Job drawing, mm, ordinate dimensions from the low corner. One solid piece. A direction names the side the tool comes from. Coordinates: 2 decimals unless noted, no trailing zeros. Order: outer loops, then holes, each group sorted by start corner. A loop starts at its lowest first (then second) coordinate and runs counter-clockwise, first axis right, second up. Notation, with made-up numbers: M -7.75,83 L 42.25,83 A27 cw 42.25,99 Z; hole C -7,76.25 d8. An arc over 180 degrees is marked long. Write item = value, one per line. Start each with the question number.
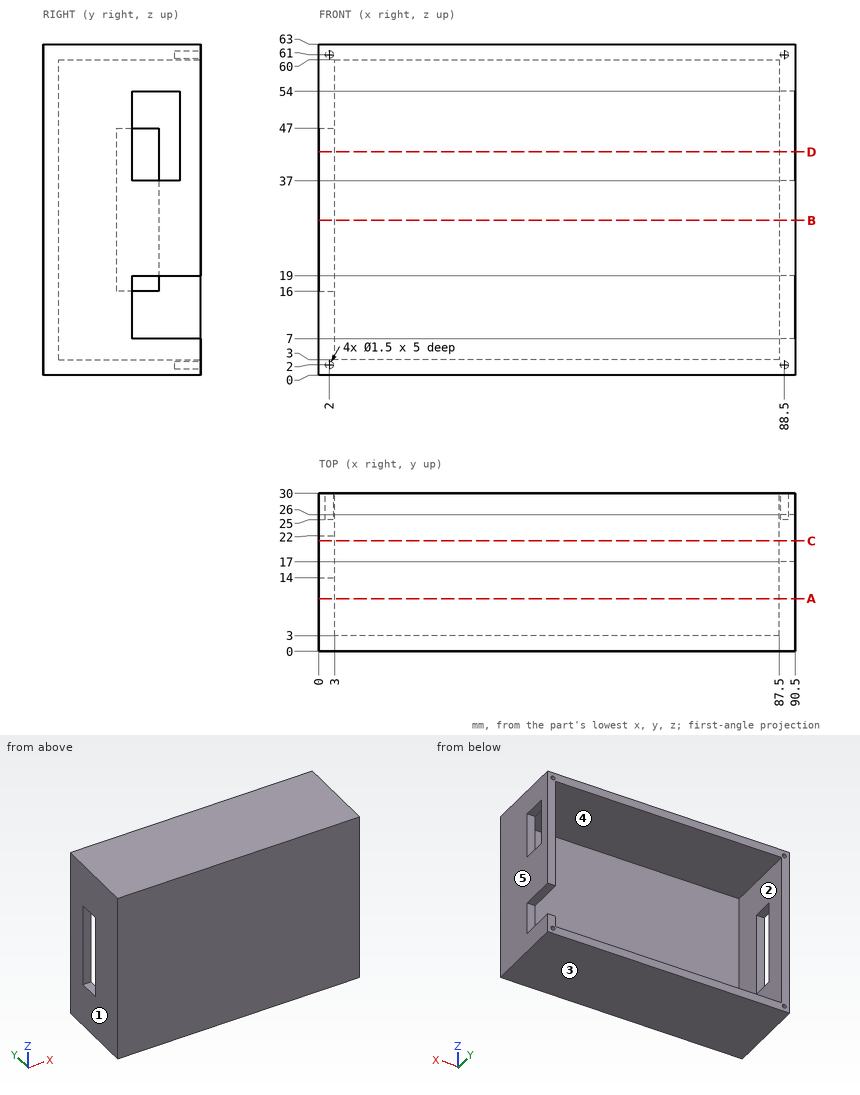
Item 1: Cut at D-D, the plane z = 42.5. Write the cut outline in (x, y).
Item 2: 3-axis set-ups, long thin cutter, end or side, ignore diameter. For the marked faces 4 and 5: which of +Z, -Z, +X, -X, +Y, -Y reach the whole face in a straight line?
Item 3: Wall check: line 1 along Z through (x, y) = (2, 27.75); line 2 along Z through (x, y) = (88.5, 26.65); line 3 along X through (y, z) = (28.85, 61). Give the ranges that are in metal, low to high. Write a range as [from, to].
Item 4: Cut at A-A, the plane y = 10. Write the cut outline in (x, z), and give its area (3 significant figures).
Item 5: Flat gauge pins, fed straight in: pin 1 (1.5 mm diameter, centred on x = 22.5, z = 24, fed in from -Y); pin 2 (1.2 mm diameter, centred on x = 2, z = 61, fed in from +Y); pin 3 (10 mm diameter, centred on x = 25, z = 43, fed in from +Y). Where does each tip first touch, or does it go through?
Item 6: Cut at B-B, the plane z = 29.5. Write the cut outline in (x, y), and give its area (4 significant figures).
Item 7: Cut at C-C, the plane y = 21. Write the cut outline in (x, z).
Item 8: Pull direction X, two halves, no side cores. Call the marked faces 1, 2 and 3: pulls with the +X half, pulls with the -X half, needs draft (parallel to the pull), parting line crosses it, or undercut.
Filled sheet:
q1.outline = M 0,0 L 90.5,0 L 90.5,17 L 87.5,17 L 87.5,3 L 3,3 L 3,14 L 0,14 Z; M 0,22 L 3,22 L 3,30 L 0,30 Z; M 87.5,26 L 90.5,26 L 90.5,30 L 87.5,30 Z
q2.face_4 = +Y
q2.face_5 = +Z, -Z, +X, +Y, -Y
q3.line_1 = [0, 1.25], [2.75, 60.25], [61.75, 63]
q3.line_2 = [0, 1.25], [2.75, 7], [19, 60.25], [61.75, 63]
q3.line_3 = [0, 1.25], [2.75, 87.75], [89.25, 90.5]
q4.outline = M 0,0 L 90.5,0 L 90.5,63 L 0,63 Z; hole M 3,3 L 87.5,3 L 87.5,60 L 3,60 Z
q4.area = 885 mm2
q5.pin_1 = 0
q5.pin_2 = 25
q5.pin_3 = 3
q6.outline = M 0,0 L 90.5,0 L 90.5,30 L 87.5,30 L 87.5,3 L 3,3 L 3,14 L 0,14 Z; M 0,22 L 3,22 L 3,30 L 0,30 Z
q6.area = 409.5 mm2
q7.outline = M 0,0 L 90.5,0 L 90.5,7 L 87.5,7 L 87.5,3 L 3,3 L 3,16 L 0,16 Z; M 0,47 L 3,47 L 3,60 L 87.5,60 L 87.5,54 L 90.5,54 L 90.5,63 L 0,63 Z; M 87.5,19 L 90.5,19 L 90.5,37 L 87.5,37 Z
q8.face_1 = pulls with the -X half
q8.face_2 = undercut
q8.face_3 = needs draft
